Check sheet for the modelled part. Datum: model origin and axes. Units: mm. Face numbers are marked on the shaded views. A direction names the side the tool comes from. Give positions to 0.01 mm unless a question says otherwise; leave off trailing zeros. Order: outer loops, then holes, each group sorted by start corner. A loop starts at its lowest first (then second) coordinate and runs counter-clockwise, first axis right, second up.
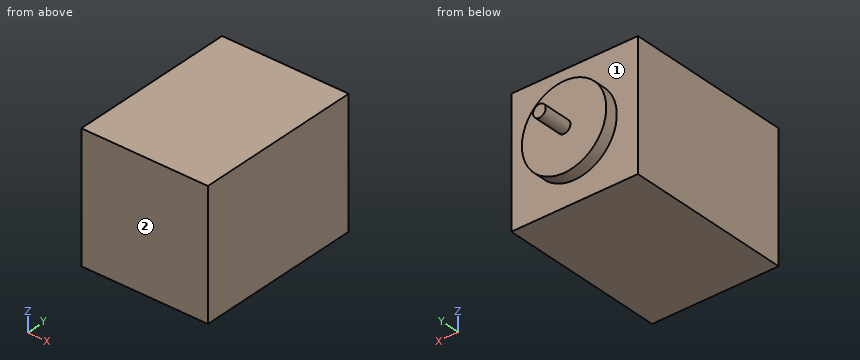
```python
from build123d import *

# Parameters (mm, degrees)
SKETCH1_W           = 30
SKETCH1_H           = 30
BOSS_EXTRUDE1_DEPTH = 40
SKETCH2_R           = 1.5
BOSS_EXTRUDE2_DEPTH = 10
SKETCH4_R           = 10
BOSS_EXTRUDE3_DEPTH = 3


with BuildPart() as part:
    # Sketch1 → Boss-Extrude1 (new body)
    with BuildSketch(Plane(origin=(0, 0, 0), x_dir=(1, 0, 0), z_dir=(0, 1, 0))):
        with Locations((15, 15)):
            Rectangle(SKETCH1_W, SKETCH1_H)
    extrude(amount=BOSS_EXTRUDE1_DEPTH)

    # Sketch2 → Boss-Extrude2 (add)
    with BuildSketch(Plane(origin=(0, 40, 0), x_dir=(1, 0, 0), z_dir=(0, 1, 0))):
        with Locations((15, 15)):
            Circle(SKETCH2_R)
    extrude(amount=BOSS_EXTRUDE2_DEPTH)

    # Sketch4 → Boss-Extrude3 (add)
    with BuildSketch(Plane(origin=(0, 40, 0), x_dir=(1, 0, 0), z_dir=(0, 1, 0))):
        with Locations((15, 15)):
            Circle(SKETCH4_R)
    extrude(amount=BOSS_EXTRUDE3_DEPTH)


solid = part.part
```
(1) Sectioned sample at C-C (z = -15). Enter the section's corners in (x, y).
(2) Sectioned sample at B-B (z = -5.75). Enter the section's corners in (x, y).
(3) Tool access check on the marked faces 1 and 2. Record the directions out of +Z, -Z, +X, -X, +Y, -Y that give a thin tool (end or side, any length) a straight path to the whole face; none if there is none.
(4) Sectioned sample at A-A (x = 15). Enter the section's corners in (y, z), plus the area to 3 significant figures.
(5) Thickness scan on L1, parallel to Y at x = 28, z = -26.75; L2, parallel to Y at x = 19, z = -23; L3, parallel to Z at x = 15, y = 42. Record the ranges inside material, lowest first.
(6) Go/stop test with flat-tipped pins: P1, Ø5, axis at y = 44, z = -26, coming from the +X side; P2, Ø8, axis at x = 20.5, z = -22.5, coming from the +Y side; P3, Ø2, axis at x = 3.5, z = -12.5, coming from the +Y side. Record where each tip stops, or that it passes through.
Values follow:
1. outline: (0, 0) - (30, 0) - (30, 40) - (25, 40) - (25, 43) - (16.5, 43) - (16.5, 50) - (13.5, 50) - (13.5, 43) - (5, 43) - (5, 40) - (0, 40) - close
2. outline: (0, 0) - (30, 0) - (30, 40) - (18.8, 40) - (18.8, 43) - (11.2, 43) - (11.2, 40) - (0, 40) - close
3. face 1: +Y
3. face 2: +Z, -Z, +X, -X, -Y
4. outline: (0, -30) - (40, -30) - (40, -25) - (43, -25) - (43, -16.5) - (50, -16.5) - (50, -13.5) - (43, -13.5) - (43, -5) - (40, -5) - (40, 0) - (0, 0) - close
4. area: 1,280 mm2
5. L1: y = 0 to 40
5. L2: y = 0 to 43
5. L3: z = -25 to -5
6. P1: stops at x = 19.92
6. P2: stops at y = 43
6. P3: stops at y = 40
